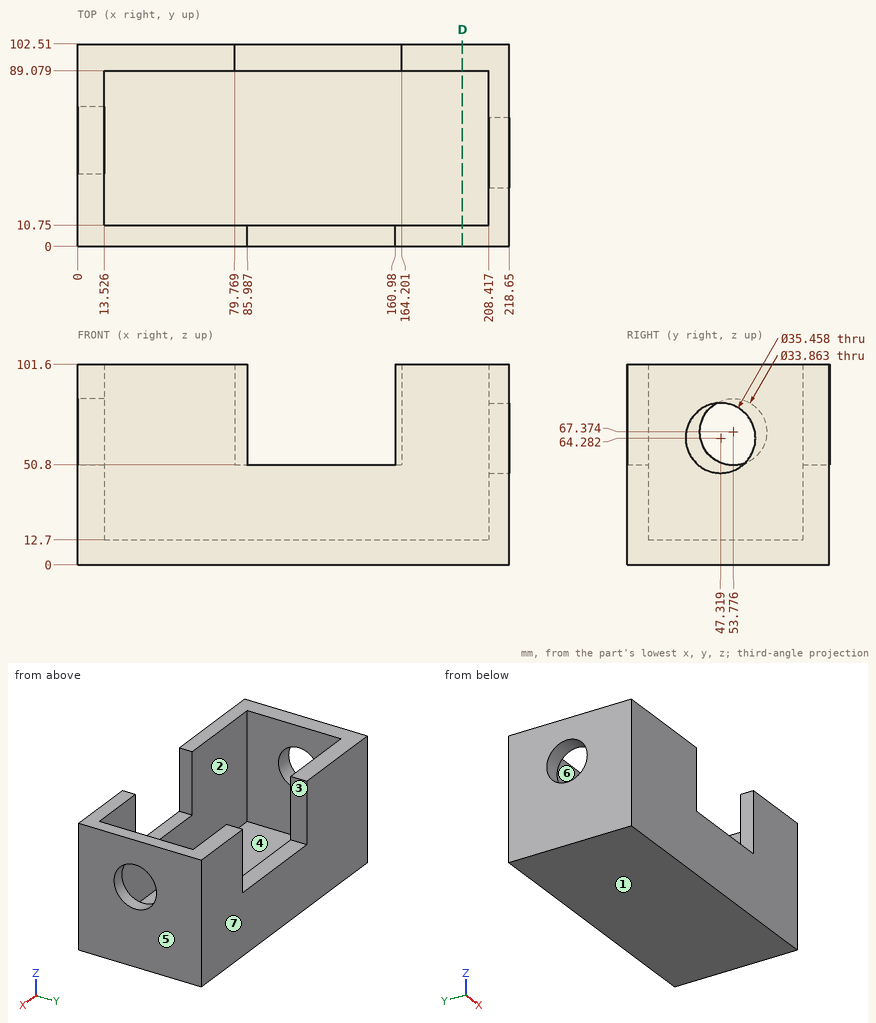
Geometry check sheet. Reference: drawing and pictorial views, mm from the part's lowest x, y, z. A direction names the side the tool comes from. Give positions to 0.01 mm unless a question says otherwise; leave off trailing zeros. Order: outer loops, then holes, each group sorted by start corner. A loop starts at its lowest first (then second) coordinate and runs counter-clockwise, first axis right, second up. Notation, with made-up numbers: M 20,73.5 L 66,73.5 A22 cw 66,101.5 Z; hole C 47,-24.5 d11. An arc over 180 degrees is marked long. Use one line per item in the form item = value. Start each with the question number.
Q1. Scan lines: line 1 along Y through (x, z) = (56, 34); line 2 along X through (y, z) = (92.5, 76); line 3 along Z through (x, y) = (130, 4.5). Record each from-to range of solid material in increasing order. Write a range as [from, to].
Q2. Access from +Z, -Z, +X, -X, +Y, -Y to the whole of each face (thin tool, end or side, straight path). Record for the marked faces 1, 2 and 3.
Q3. Mould release check, pull along X, two halves, no side actions. Record for the marked faces 4, 5, 6 and 7: +X half, -X half, draft (parallel to the pull), parting line (faces both ways), or undercut.
Q4. Section check D-D (x = 195). Enter the section's corners in (y, z).
Q5. Go/stop test with flat-tipped pins: pin 1 Ø10.5 at (x, y) = (109, 96) entering from +Z; pin 2 Ø23.5 at (x, y) = (82.5, 41) entering from +Z. Record where each tip stops, or that it passes through.
Evaluation:
q1.line_1 = [0, 10.75], [89.08, 102.51]
q1.line_2 = [0, 79.77], [164.2, 218.65]
q1.line_3 = [0, 50.8]
q2.face_1 = -Z, +X, -X, +Y, -Y
q2.face_2 = +Z
q2.face_3 = +Z, +Y
q3.face_4 = undercut
q3.face_5 = +X half
q3.face_6 = undercut
q3.face_7 = draft
q4.outline = M 0,0 L 102.51,0 L 102.51,101.6 L 89.08,101.6 L 89.08,12.7 L 10.75,12.7 L 10.75,101.6 L 0,101.6 Z
q5.pin_1 = 50.8
q5.pin_2 = 12.7
